from build123d import *

# Parameters (mm, degrees)
SKETCH1_W           = 9
SKETCH1_H           = 6
BOSS_EXTRUDE1_DEPTH = 5
SKETCH3_R           = 1.25
CUT_EXTRUDE2_DEPTH  = 4
SKETCH2_R           = 0.795
CUT_EXTRUDE1_DEPTH  = 1
CUT_EXTRUDE3_DEPTH  = 6


with BuildPart() as part:
    # Sketch1 → Boss-Extrude1 (new body)
    with BuildSketch(Plane(origin=(0, 0, 0), x_dir=(1, 0, 0), z_dir=(0, 1, 0))):
        Rectangle(SKETCH1_W, SKETCH1_H)
    extrude(amount=BOSS_EXTRUDE1_DEPTH)

    # Sketch3 → Cut-Extrude2 (cut)
    with BuildSketch(Plane.XZ):
        with Locations((-1.5, 0)):
            Circle(SKETCH3_R)
    extrude(amount=-CUT_EXTRUDE2_DEPTH, mode=Mode.SUBTRACT)

    # Sketch2 → Cut-Extrude1 (cut)
    with BuildSketch(Plane.XZ):
        with Locations((-3.25, -1.875)):
            Circle(SKETCH2_R)
        with Locations((-3.25, 1.875)):
            Circle(SKETCH2_R)
        with Locations((1.5, 0)):
            Circle(SKETCH2_R)
    extrude(amount=-CUT_EXTRUDE1_DEPTH, mode=Mode.SUBTRACT)

    # Sketch4 → Cut-Extrude3 (cut, through all)
    with BuildSketch(Plane.XZ):
        Polygon((3.839906766, -3), (4.5, -2.00986015), (4.5, -3), align=None)
    extrude(amount=-CUT_EXTRUDE3_DEPTH, mode=Mode.SUBTRACT)


solid = part.part
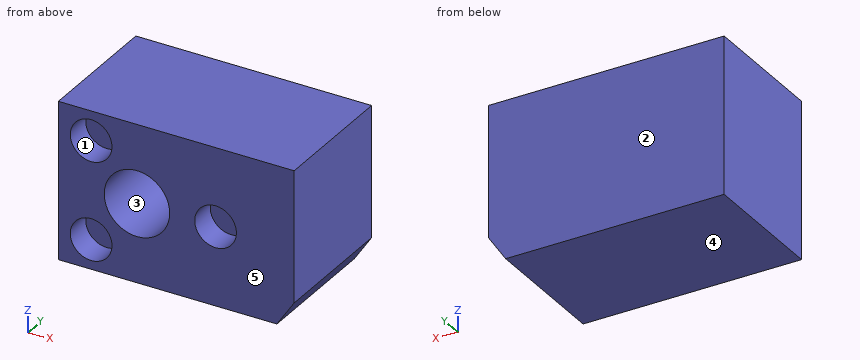
The listing builds one solid part. Answer for the finished solid, in the listing's coordinates (mm). Face numbers are marked on the shaded views. A direction names the side the tool comes from. Give positions to 0.01 mm unless a question says otherwise; leave off trailing zeros. Write each loop counter-clockwise with the first axis right and the second up, starting at its lowest first coordinate (ties: lowest second). Pieces come first, ordered by that corner, then holes. Notation, with made-up numbers: (-29.5, 71) -> (-1.5, 71) arc R29 cw to (-1.5, 92) -> close; hole circle Ø4 at (87, -15). An arc over 180 degrees is marked (long way). One line per question, with ' | ' between items. Start each with the question number.
1. Section B-B (x = -0.5) is taken. Determine the outline of the cut face in (y, z), plus the area to 3 significant figures.
2. For a pull along Z with two mould halves and no side action, classify the marked faces 3, 4 and 5 as pulls with the +Z half, pulls with the -Z half, needs draft (parallel to the pull), parting line crosses it, or undercut.
3. Given pin 1 Ø0.8 at (x, z) = (-1.5, 0.5) entering from -Y, flat-ended and moving along its own axis, determine where the tip first touches the part or whether it passes through.
4. Section D-D (x = -3.25) is taken. Determine the outline of the cut face in (y, z), plus the area to 3 significant figures.
5. Find the intervals of material crossed by probe 1 along Z at (x, y) = (-3.25, 0.35); probe 2 along Z at (x, y) = (1.5, 0.75) (3 decimals); probe 3 along Y at (x, z) = (2, -0.15), in increasing order.
6. Section C-C (z = 2.4) is taken. Determine the outline of the cut face in (x, y).
7. Section A-A (y = 2.8) is taken. Determine the outline of the cut face in (x, z), plus the area to 3 significant figures.
8. For the marked faces 1 and 2, determine the directions among +Z, -Z, +X, -X, +Y, -Y from which every point of the face is accessible in a straight line to the end or side of a thin tool.
Response values:
1) outline: (0, -3) -> (5, -3) -> (5, 3) -> (0, 3) -> (0, 0.75) -> (4, 0.75) -> (4, -0.75) -> (0, -0.75) -> close | area: 24.0 mm2
2) face 3: undercut | face 4: pulls with the -Z half | face 5: needs draft
3) pin 1: y = 4
4) outline: (0, -3) -> (5, -3) -> (5, 3) -> (0, 3) -> (0, 2.67) -> (1, 2.67) -> (1, 1.08) -> (0, 1.08) -> (0, -1.08) -> (1, -1.08) -> (1, -2.67) -> (0, -2.67) -> close | area: 26.8 mm2
5) probe 1: -3 to -2.67, -1.08 to 1.08, 2.67 to 3 | probe 2: -3 to -0.795, 0.795 to 3 | probe 3: 1 to 5
6) outline: (-4.5, 0) -> (-3.85, 0) -> (-3.85, 1) -> (-2.65, 1) -> (-2.65, 0) -> (4.5, 0) -> (4.5, 5) -> (-4.5, 5) -> close
7) outline: (-4.5, -3) -> (3.84, -3) -> (4.5, -2.01) -> (4.5, 3) -> (-4.5, 3) -> close; hole circle Ø2.5 at (-1.5, 0) | area: 48.8 mm2
8) face 1: -Y | face 2: +Z, -Z, +X, -X, +Y
